The listing builds one solid part. Answer for the finished solid, in the listing's coordinates (mm). Give positions to 0.01 mm unless a question says otherwise; leave off trailing zeros. Order: outer loops, then holes, each group sorted by start corner. A loop starts at its lowest first (then second) coordinate and runs counter-clockwise, first axis right, second up. Notation, with made-up numbers: (21, 73.25) - (69, 73.25) arc R24 cw to (69, 93.25) - close; hole circle Ø8 at (-2, 54). An arc over 180 degrees is marked (long way). Answer as CSV lines item,"result". Start each with the question number.
1. Section A-A on z = 303.5 is taken. Give the vertices of the cut face in (x, y), and give its area (3 significant figures).
2. A flat-ended cylindrical pin translates along its axis: pin 1 (4.5 mm diameter, centred on x = 5.5, z = 185, fed in from +Y). Find the tip coordinate at first contact, or state that the pin passes through.
3. Consider line 1 along Y through (x, z) = (0.25, 191); line 2 along X through (y, z) = (4, 60); line 3 along X through (y, z) = (7.5, 324). Determine where each line is inside the solid, lowest interval first. Write a range as [from, to].
Autodesk Inventor part; units mm, degrees
ref_plane "YZ Plane" through (0, 0, 0) normal (1, 0, 0) x (0, 1, 0)
ref_plane "XZ Plane" through (0, 0, 0) normal (0, 1, 0) x (-1, 0, 0)
ref_plane "XY Plane" through (0, 0, 0) normal (0, 0, 1) x (1, 0, 0)
sketch "Szkic1" plane through (0, 0, 0) normal (0, 0, 1) x (1, 0, 0)
  line L0 (-0.5, 7.4119) -> (0, 8)
  line L1 (-0.5, 6.5901) -> (-0.5, 7.4119)
  arc A0 (0.0193, 6.0131) -> (-0.4182, 6.4505) centre (-0.9753, 5.4559) ccw
  arc A1 (-0.5, 6.5901) -> (-0.4182, 6.4505) centre (-0.34, 6.5901) ccw
  arc A2 (0.0193, 6.0131) -> (0.1589, 5.9313) centre (0.1589, 6.0913) ccw
  line L2 (0.5806, 5.9313) -> (0.1589, 5.9313)
  arc A3 (0.5806, 4.9806) -> (0.5806, 5.9313) centre (0.7358, 5.4559) ccw
  line L3 (0.1589, 4.9806) -> (0.5806, 4.9806)
  arc A4 (-0.4182, 4.4613) -> (0.0193, 4.8988) centre (-0.9753, 5.4559) ccw
  arc A5 (0.1589, 4.9806) -> (0.0193, 4.8988) centre (0.1589, 4.8206) ccw
  arc A6 (-0.4182, 4.4613) -> (-0.5, 4.3217) centre (-0.34, 4.3217) ccw
  line L4 (-0.5, 0.5) -> (-0.5, 4.3217)
  line L5 (0, 0) -> (-0.5, 0.5)
  line L6 (11, 0) -> (0, 0)
  line L7 (11.5, 0.5) -> (11, 0)
  line L8 (11.5, 4.3217) -> (11.5, 0.5)
  arc A7 (11.5, 4.3217) -> (11.4182, 4.4613) centre (11.34, 4.3217) ccw
  arc A8 (10.9807, 4.8988) -> (11.4182, 4.4613) centre (11.9753, 5.4559) ccw
  arc A9 (10.9807, 4.8988) -> (10.8411, 4.9806) centre (10.8411, 4.8206) ccw
  line L9 (10.4194, 4.9806) -> (10.8411, 4.9806)
  arc A10 (10.4194, 5.9313) -> (10.4194, 4.9806) centre (10.2642, 5.4559) ccw
  line L10 (10.8411, 5.9313) -> (10.4194, 5.9313)
  arc A11 (10.8411, 5.9313) -> (10.9807, 6.0131) centre (10.8411, 6.0913) ccw
  arc A12 (11.4182, 6.4505) -> (10.9807, 6.0131) centre (11.9753, 5.4559) ccw
  line L11 (11.5, 7.4119) -> (11.5, 6.5901)
  arc A13 (11.4182, 6.4505) -> (11.5, 6.5901) centre (11.34, 6.5901) ccw
  line L12 (11, 8) -> (11.5, 7.4119)
  line L13 (0, 8) -> (11, 8)
extrude "Wyciągnięcie proste1" add sketch "Szkic1" along normal blind 407
sketch "Szkic2" plane through (0, 8, 0) normal (0, 1, 0) x (1, 0, 0)
  line L0 (11, 0) -> (11, -407)
  line L1 (0, 0) -> (0, -407)
  line L2 (0, 0) -> (11, 0)
  line L3 (0, 0) -> (0, -407)
  line L4 (11, -407) -> (0, -407)
  line L5 (11, 0) -> (11, -407)
  point P0 (5.5, -10)
  point P1 (5.5, -35)
  point P2 (5.5, -60)
  point P3 (5.5, -85)
  point P4 (5.5, -110)
  point P5 (5.5, -135)
  point P6 (5.5, -160)
  point P7 (5.5, -185)
  point P8 (5.5, -210)
  point P9 (5.5, -235)
  point P10 (5.5, -260)
  point P11 (5.5, -285)
  point P12 (5.5, -310)
  point P13 (5.5, -335)
  point P14 (5.5, -360)
  point P15 (5.5, -385)
  dimension "d2" = 11
  dimension "d3" = 5.5
  dimension "d4" = 10
  dimension "d7" = 25
hole "Otwór1" at (5.5, 8, 10) at (5.5, 8, 35) at (5.5, 8, 60) at (5.5, 8, 85) at (5.5, 8, 110) at (5.5, 8, 135) at (5.5, 8, 160) at (5.5, 8, 185) at (5.5, 8, 210) at (5.5, 8, 235) at (5.5, 8, 260) at (5.5, 8, 285) at (5.5, 8, 310) at (5.5, 8, 335) at (5.5, 8, 360) at (5.5, 8, 385) direction (0, -1, 0) diameter 3.5 end through all
hole "Otwór2" at (5.5, 8, 210) at (5.5, 8, 385) at (5.5, 8, 360) at (5.5, 8, 335) at (5.5, 8, 310) at (5.5, 8, 285) at (5.5, 8, 260) at (5.5, 8, 235) at (5.5, 8, 185) at (5.5, 8, 160) at (5.5, 8, 135) at (5.5, 8, 110) at (5.5, 8, 85) at (5.5, 8, 60) at (5.5, 8, 35) at (5.5, 8, 10) direction (0, -1, 0) diameter 6 depth 4.6
properties part number "COTS_HIWIN_MGN12_RAIL_407mm"
Checks:
1,outline,"(-0.5, 0.5) - (0, 0) - (11, 0) - (11.5, 0.5) - (11.5, 4.32) arc R0.16 ccw to (11.42, 4.46) arc R1.14 cw to (10.98, 4.9) arc R0.16 ccw to (10.84, 4.98) - (10.42, 4.98) arc R0.5 cw (long way) to (10.42, 5.93) - (10.84, 5.93) arc R0.16 ccw to (10.98, 6.01) arc R1.14 cw to (11.42, 6.45) arc R0.16 ccw to (11.5, 6.59) - (11.5, 7.41) - (11, 8) - (0, 8) - (-0.5, 7.41) - (-0.5, 6.59) arc R0.16 ccw to (-0.42, 6.45) arc R1.14 cw to (0.02, 6.01) arc R0.16 ccw to (0.16, 5.93) - (0.58, 5.93) arc R0.5 cw (long way) to (0.58, 4.98) - (0.16, 4.98) arc R0.16 ccw to (0.02, 4.9) arc R1.14 cw to (-0.42, 4.46) arc R0.16 ccw to (-0.5, 4.32) - close"
1,area,"91.5 mm²"
2,pin 1,"stops at y = 3.4"
3,line 1,"y = [0, 4.98], [5.93, 8]"
3,line 2,"x = [-0.5, 2.5], [8.5, 11.5]"
3,line 3,"x = [-0.43, 11.43]"
